from build123d import *

# Parameters (mm, degrees)
SKETCH1_W           = 25.4
SKETCH1_H           = 86.36
SKETCH1_R           = 2.032
SKETCH1_R_2         = 4
SKETCH1_R_3         = 4.669733183
BOSS_EXTRUDE1_DEPTH = 3.175
FILLET1_R           = 3.81


with BuildPart() as part:
    # Sketch1 → Boss-Extrude1 (new body)
    with BuildSketch(Plane(origin=(0, 0, 0), x_dir=(1, 0, 0), z_dir=(0, 1, 0))):
        Rectangle(SKETCH1_W, SKETCH1_H)
        with Locations(Location((-6.35, -29.21, 0), (0, 0, 270))):
            Circle(SKETCH1_R, mode=Mode.SUBTRACT)
        with Locations(Location((6.35, -29.21, 0), (0, 0, 270))):
            Circle(SKETCH1_R, mode=Mode.SUBTRACT)
        with Locations(Location((0, -5.08, 0), (0, 0, 270))):
            Circle(SKETCH1_R_2, mode=Mode.SUBTRACT)
        with Locations(Location((0, 26.67, 0), (0, 0, 270))):
            Circle(SKETCH1_R_3, mode=Mode.SUBTRACT)
    extrude(amount=BOSS_EXTRUDE1_DEPTH)

    # Fillet1
    fillet1_edges = [part.edges().sort_by_distance(p)[0] for p in [
        (-12.7, 1.5875, 43.18),
        (-12.7, 1.5875, -43.18),
        (12.7, 1.5875, -43.18),
        (12.7, 1.5875, 43.18),
    ]]
    fillet(fillet1_edges, radius=FILLET1_R)


solid = part.part
Model file for the job. Use its own axes, mm. Coordinates: 2 decimals unless noted, no trailing zeros. Write each loop counter-clockwise with the first axis right and the second up, starting at its lowest first coordinate (ties: lowest second). Pieces come first, ordered by that corner, then holes. Notation, with made-up numbers: (11.25, -23) - (51.25, -23) arc R15 cw to (51.25, -16) - close; hole circle Ø7 at (-35.5, 76). An arc over 180 degrees is marked (long way). Write each question's results on one line, items separated by ' | '. Start each with the question number.
1) Mould opens along Z. For faces 1 (the face through (0, 0, -1)), 2 (the face through (11.554, 1.61, -42.094)), 3 (the face through (1.403, 1.565, -22.216)), 4 (the face through (6.96, 1.57, 31.15)) say: pulls with the +Z half, pulls with the -Z half, needs draft (parallel to the pull), parting line crosses it, or undercut.
2) Cut at D-D (z = -26.67). Write the cut outline in (x, y) (3 decimals).
3) Cut at A-A (z = 29.21). Write the cut outline in (x, y) (3 decimals).
4) Flat gauge pin, fed straight in: P1, Ø3.5, axis at x = -6.35, z = 29.21, coming from the -Y side. Where does the tip first touch, or does it go through?
5) Probe line 1 along X through (y, z) = (2.45, 29.21); line 2 along X through (y, z) = (1.45, -26.67); line 3 along X through (y, z) = (1.8, 5.08). List the from-to ranges inside material, lowest first. Write a range as from..to.
6) Cut at C-C (y = 1). Write the cut outline in (x, z), then the cut area to 3 significant figures.
7) Cut at B-B (x = 0). Write the cut outline in (y, z) (3 decimals).
Returned:
1) face 1: needs draft | face 2: pulls with the -Z half | face 3: undercut | face 4: undercut
2) outline: (-12.7, 0) - (-4.67, 0) - (-4.67, 3.175) - (-12.7, 3.175) - close; (4.67, 0) - (12.7, 0) - (12.7, 3.175) - (4.67, 3.175) - close
3) outline: (-12.7, 0) - (-8.382, 0) - (-8.382, 3.175) - (-12.7, 3.175) - close; (-4.318, 0) - (4.318, 0) - (4.318, 3.175) - (-4.318, 3.175) - close; (8.382, 0) - (12.7, 0) - (12.7, 3.175) - (8.382, 3.175) - close
4) P1: through
5) line 1: -12.7..-8.38, -4.32..4.32, 8.38..12.7 | line 2: -12.7..-4.67, 4.67..12.7 | line 3: -12.7..-4, 4..12.7
6) outline: (-12.7, -39.37) arc R3.81 ccw to (-8.89, -43.18) - (8.89, -43.18) arc R3.81 ccw to (12.7, -39.37) - (12.7, 39.37) arc R3.81 ccw to (8.89, 43.18) - (-8.89, 43.18) arc R3.81 ccw to (-12.7, 39.37) - close; hole circle Ø4.06 at (-6.35, 29.21); hole circle Ø9.34 at (0, -26.67); hole circle Ø8 at (0, 5.08); hole circle Ø4.06 at (6.35, 29.21) | area: 2,040 mm^2
7) outline: (0, -43.18) - (3.175, -43.18) - (3.175, -31.34) - (0, -31.34) - close; (0, -22) - (3.175, -22) - (3.175, 1.08) - (0, 1.08) - close; (0, 9.08) - (3.175, 9.08) - (3.175, 43.18) - (0, 43.18) - close
